from build123d import *

# Parameters (mm, degrees)
SKETCH2_W           = 30
SKETCH2_H           = 30
SKETCH2_R           = 6.2
BOSS_EXTRUDE2_DEPTH = 30
SKETCH4_W           = 6
SKETCH4_H           = 30
BOSS_EXTRUDE3_DEPTH = 30
FILLET1_R           = 8
FILLET4_R           = 10
SKETCH5_R           = 6
CUT_EXTRUDE1_DEPTH  = 30
FILLET5_R           = 6


with BuildPart() as part:
    # Sketch2 → Boss-Extrude2 (new body)
    with BuildSketch(Plane.XY):
        Rectangle(SKETCH2_W, SKETCH2_H)
        Circle(SKETCH2_R, mode=Mode.SUBTRACT)
    extrude(amount=BOSS_EXTRUDE2_DEPTH)

    # Sketch4 → Boss-Extrude3 (add)
    with BuildSketch(Plane(origin=(0, 15, 0), x_dir=(1, 0, 0), z_dir=(0, 1, 0))):
        with Locations((-12, -15)):
            Rectangle(SKETCH4_W, SKETCH4_H)
        with Locations((12, -15)):
            Rectangle(SKETCH4_W, SKETCH4_H)
    extrude(amount=BOSS_EXTRUDE3_DEPTH)

    # Fillet1
    fillet1_edges = [part.edges().sort_by_distance(p)[0] for p in [
        (15, -15, 15),
        (-15, -15, 15),
    ]]
    fillet(fillet1_edges, radius=FILLET1_R)

    # Fillet4
    fillet4_edges = [part.edges().sort_by_distance(p)[0] for p in [
        (-12, 45, 30),
        (-12, 45, 0),
        (12, 45, 30),
        (12, 45, 0),
    ]]
    fillet(fillet4_edges, radius=FILLET4_R)

    # Sketch5 → Cut-Extrude1 (cut)
    with BuildSketch(Plane.ZY.offset(15)):
        with Locations(Location((15, 35, 0), (0, 0, 270))):
            Circle(SKETCH5_R)
    extrude(amount=-CUT_EXTRUDE1_DEPTH, mode=Mode.SUBTRACT)

    # Fillet5
    fillet5_edges = [part.edges().sort_by_distance(p)[0] for p in [
        (-9, 15, 15),
        (9, 15, 15),
    ]]
    fillet(fillet5_edges, radius=FILLET5_R)


solid = part.part
Work out the finished part from the listing and answer in its coordinate system (mm). A direction names the side the tool comes from. Round coordinates to 2 decimals unless told otherwise and drop trailing zeros. Write each loop counter-clockwise with the first axis right and the second up, starting at its lowest first coordinate (ties: lowest second). Pieces come first, ordered by that corner, then holes.
1) A cutting plane is placed at B-B (x = 0). Give the vertices of the cut face in (y, z), plus the area to 3 significant figures.
2) A cutting plane is placed at D-D (z = 26). Give the vertices of the cut face in (x, y).
3) A cutting plane is placed at A-A (z = 15). Give the vertices of the cut face in (x, y).
4) Straight lines are drawn through the part: line 1 (X direction, y = 27.5, z = 14.5); line 2 (Y direction, x = 0, z = 6.25); line 3 (Z direction, x = 10.25, y = 35). For each, find the intervals that lie inside material, in ascending order.
5) Given pin 1 Ø6.5 at (x, z) = (0, 8.5) entering from +Y; pin 2 Ø11 at (y, z) = (35, 15) entering from -X; pin 3 Ø2 at (x, z) = (3.5, 22) entering from +Y, each flat-ended and moving along its own axis, determine where each tip first touches the part or whether it passes through.
6) The mould has two halves that part along Z. Classify faces 3 (the cylindrical face through (-7.289, 16.804, 14.79)), 4 (the cylindrical face through (12.04, 41.99, 2.85)), 5 (the cylindrical face through (12, 41, 15)): pulls with the +Z half, pulls with the -Z half, needs draft (parallel to the pull), parting line crosses it, or undercut.
7) A cutting plane is placed at C-C (y = 22). Give the vertices of the cut face in (x, z), plus the area to 3 significant figures.
8) A tool of negligible diameter and unlimited length cuts with its end or side. For faces 1 (the flat face through (9, 27, 15)), 2 (the flat face through (15, 19, 15)), from which of +Z, -Z, +X, -X, +Y, -Y can it reach the whole face along a straight path? Write none if from no direction.
Completed:
1. outline: (-15, 0) - (-6.2, 0) - (-6.2, 30) - (-15, 30) - close; (6.2, 0) - (15, 0) - (15, 30) - (6.2, 30) - close
1. area: 528 mm2
2. outline: (-15, -7) arc R8 ccw to (-7, -15) - (7, -15) arc R8 ccw to (15, -7) - (15, 43) - (9, 43) - (9, 21) arc R6 cw to (3, 15) - (-3, 15) arc R6 cw to (-9, 21) - (-9, 43) - (-15, 43) - close; hole circle Ø12.4 at (0, 0)
3. outline: (-15, -7) arc R8 ccw to (-7, -15) - (7, -15) arc R8 ccw to (15, -7) - (15, 29) - (9, 29) - (9, 21) arc R6 cw to (3, 15) - (-3, 15) arc R6 cw to (-9, 21) - (-9, 29) - (-15, 29) - close; (-15, 41) - (-9, 41) - (-9, 45) - (-15, 45) - close; (9, 41) - (15, 41) - (15, 45) - (9, 45) - close; hole circle Ø12.4 at (0, 0)
4. line 1: x = -15 to -9, 9 to 15
4. line 2: y = -15 to -6.2, 6.2 to 15
4. line 3: z = 0 to 9, 21 to 30
5. pin 1: stops at y = 15.01
5. pin 2: passes through
5. pin 3: stops at y = 15.19
6. face 3: needs draft
6. face 4: pulls with the -Z half
6. face 5: undercut
7. outline: (-15, 0) - (-9, 0) - (-9, 30) - (-15, 30) - close; (9, 0) - (15, 0) - (15, 30) - (9, 30) - close
7. area: 360 mm2
8. face 1: +Z, -Z, +Y
8. face 2: +Z, -Z, +X, +Y, -Y
